Part model, mm, in its own coordinate system. Give positions to 0.01 mm unless a question says otherwise; leave off trailing zeros. Write each loop counter-clockwise with the first axis right and the second up, starting at its lowest first coordinate (ties: lowest second). Pieces come first, ordered by that corner, then holes.
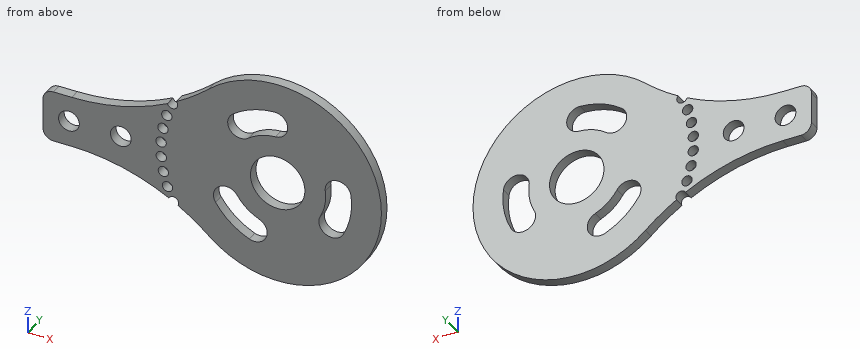
```python
from build123d import *

# Parameters (mm, degrees)
EXTRUDE_1_DEPTH          = 2
SKETCH_2_R               = 1
CUT_EXTRUDE_1_DEPTH      = 3
PATTERN_CIRCULAR_1_COUNT = 8
PATTERN_CIRCULAR_1_ANGLE = 52.5
SKETCH_3_R               = 2
CUT_EXTRUDE_2_DEPTH      = 3
PATTERN_LINEAR_1_COUNT   = 2
PATTERN_LINEAR_1_PITCH   = 10
CUT_EXTRUDE_4_DEPTH      = 3
PATTERN_CIRCULAR_3_COUNT = 3
SKETCH_7_R               = 5.25
CUT_EXTRUDE_5_DEPTH      = 3


with BuildPart() as part:
    # Эскиз1 → Бобышка-Вытянуть1 (new body)
    with BuildSketch(Plane(origin=(0, 0, 0), x_dir=(1, 0, 0), z_dir=(0, 1, 0))):
        with BuildLine():
            Line((0, -2), (0, -8))
            ThreePointArc((0, -8), (0.585786438, -9.414213562), (2, -10))
            Line((2, -10), (5.542486889, -10))
            ThreePointArc((5.542486889, -10), (19.684622513, -12.583426132), (32, -20))
            ThreePointArc((32, -20), (65.228756555, -5), (32, 10))
            ThreePointArc((32, 10), (19.684622513, 2.583426132), (5.542486889, 0))
            Line((5.542486889, 0), (2, 0))
            ThreePointArc((2, 0), (0.585786438, -0.585786438), (0, -2))
        make_face()
    extrude(amount=EXTRUDE_1_DEPTH)

    # Эскиз2 → Вырез-Вытянуть1 (cut, through all)
    with BuildSketch(Plane(origin=(0, 2, 0), x_dir=(1, 0, 0), z_dir=(0, 1, 0))):
        with Locations((25.137189268, 5.128125392)):
            Circle(SKETCH_2_R)
    cut_extrude_1 = extrude(amount=-CUT_EXTRUDE_1_DEPTH, mode=Mode.SUBTRACT)

    # Круговой массив1: Вырез-Вытянуть1 ×8 about axis
    pattern_circular_1_axis = Axis((45.228756555, 0, 5), (0, 1, 0))
    for i in range(1, PATTERN_CIRCULAR_1_COUNT):
        add(cut_extrude_1.rotate(pattern_circular_1_axis, i * PATTERN_CIRCULAR_1_ANGLE / (PATTERN_CIRCULAR_1_COUNT - 1)), mode=Mode.SUBTRACT)

    # Эскиз3 → Вырез-Вытянуть2 (cut, through all)
    with BuildSketch(Plane(origin=(0, 2, 0), x_dir=(1, 0, 0), z_dir=(0, 1, 0))):
        with Locations((5, -5)):
            Circle(SKETCH_3_R)
    cut_extrude_2 = extrude(amount=-CUT_EXTRUDE_2_DEPTH, mode=Mode.SUBTRACT)

    # Линейный массив1: Вырез-Вытянуть2 ×2
    with Locations(*[(i * PATTERN_LINEAR_1_PITCH, 0, 0) for i in range(1, PATTERN_LINEAR_1_COUNT)]):
        add(cut_extrude_2, mode=Mode.SUBTRACT)

    # Эскиз6 → Вырез-Вытянуть4 (cut, through all)
    with BuildSketch(Plane(origin=(0, 2, 0), x_dir=(1, 0, 0), z_dir=(0, 1, 0))):
        with BuildLine():
            ThreePointArc((37.446222009, -0.000750623), (39.288664725, 2.090532233), (41.67041088, 3.538062681))
            ThreePointArc((41.67041088, 3.538062681), (43.016297342, 6.807403537), (39.746956487, 8.153289999))
            ThreePointArc((39.746956487, 8.153289999), (36.077763715, 5.923300776), (33.239393437, 2.701580475))
            ThreePointArc((33.239393437, 2.701580475), (33.991642174, -0.75299936), (37.446222009, -0.000750623))
        make_face()
    cut_extrude_4 = extrude(amount=-CUT_EXTRUDE_4_DEPTH, mode=Mode.SUBTRACT)

    # Круговой массив3: Вырез-Вытянуть4 ×3 about axis
    pattern_circular_3_axis = Axis((45.228756555, 0, 5), (0, 1, 0))
    for i in range(1, PATTERN_CIRCULAR_3_COUNT):
        add(cut_extrude_4.rotate(pattern_circular_3_axis, i * 360 / PATTERN_CIRCULAR_3_COUNT), mode=Mode.SUBTRACT)

    # Эскиз7 → Вырез-Вытянуть5 (cut, through all)
    with BuildSketch(Plane(origin=(0, 2, 0), x_dir=(1, 0, 0), z_dir=(0, 1, 0))):
        with Locations((45.228756555, -5)):
            Circle(SKETCH_7_R)
    extrude(amount=-CUT_EXTRUDE_5_DEPTH, mode=Mode.SUBTRACT)


solid = part.part
```
1) Saw through at C-C, the plane x = 34.5. Write the cut outline in (y, z), then the cut area to 3 significant figures.
Answers follow:
outline: (0, -11.88) - (2, -11.88) - (2, -4.38) - (0, -4.38) - close; (0, 1) - (2, 1) - (2, 21.88) - (0, 21.88) - close
area: 56.8 mm2
2) Pin check, flat tip, straight feed: pin 1 Ø1.6 at (x, z) = (23.2, 0.42) entering from -Y. Stop position of the tip, or through.
Answers follow:
pin 1: passes through
3) Wall check: L1, parallel to X at y = 0.9, z = 5; L2, parallel to Z at x = 5, y = 1.8; L3, parallel to Z at x = 38.5, y = 0.7. Give the ranges that are in metal, low to high.
Answers follow:
L1: x = 0 to 3, 7 to 13, 17 to 39.98, 50.48 to 54.48, 59.48 to 65.23
L2: z = 0 to 3, 7 to 10
L3: z = -13.83 to -7.56, -1.35 to 11.87, 17.56 to 23.83
4) Saw through at A-A, the plane x = 15. Write the cut outline in (y, z), then the cut area to 3 significant figures.
Answers follow:
outline: (0, -1.13) - (2, -1.13) - (2, 3) - (0, 3) - close; (0, 7) - (2, 7) - (2, 11.13) - (0, 11.13) - close
area: 16.5 mm2
5) Saw through at B-B, the plane y = 0.3. Count the separate pieces of the cut face and the enclosed holes in it, then the cut area to 3 significant figures.
Answers follow:
separate pieces: 1
enclosed holes: 12
area: 1,300 mm2
